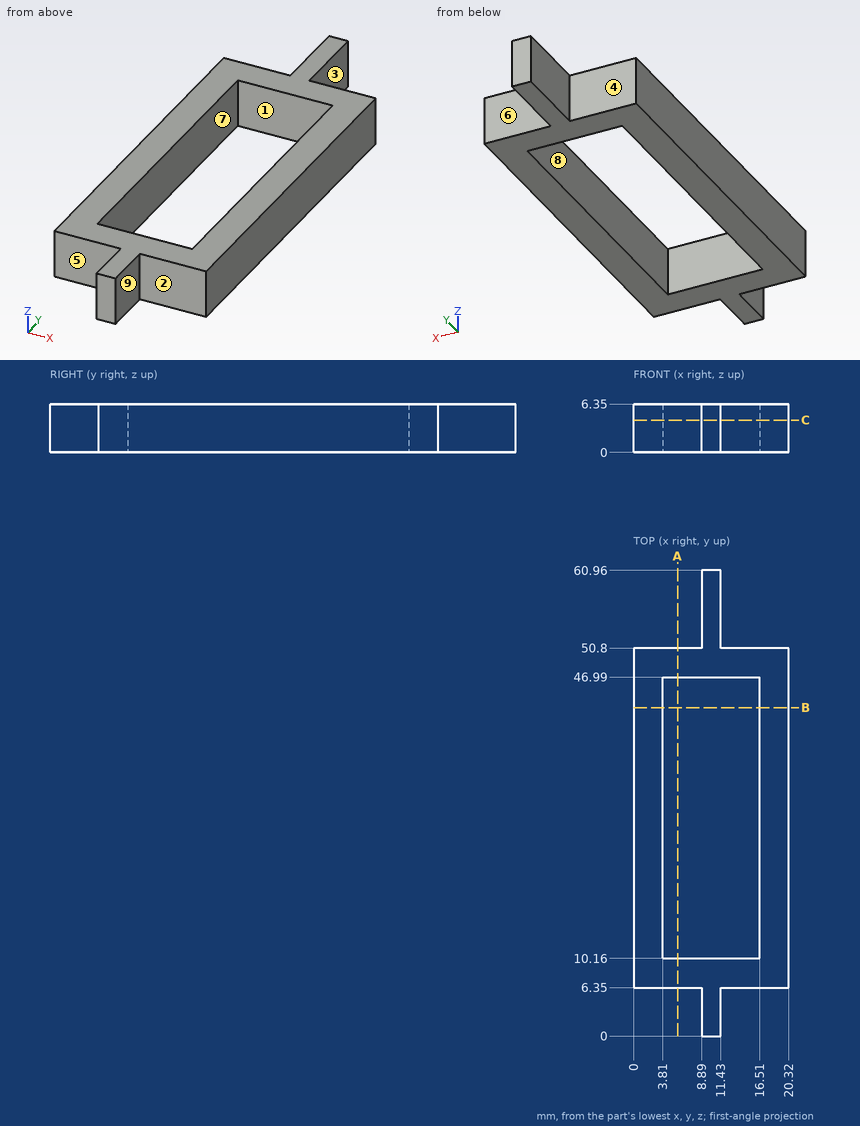
Drawing for the job (mm, zero at the part's lowest x, y, z). A direction names the side the tool comes from. Round coordinates to 2 decimals unless told otherwise and drop trailing zeros. Loops run counter-clockwise (first coordinate to the right, second up) from the corner with the lowest first, then second, coordinate; pieces in that order, holes last. Notation, with made-up numbers: (40, -33.75) -> (44, -33.75) arc R15 cw to (44, -7.75) -> close; hole circle Ø1 at (26.25, 36.5). An arc over 180 degrees is marked (long way). Answer in a Markdown table with one row per item.
Item 1: Saw through at A-A (x = 5.75). Write the cut outline in (y, z), and give its area (3 significant figures).
Answers below:
| item | result |
|---|---|
| outline | (6.35, 0) -> (10.16, 0) -> (10.16, 6.35) -> (6.35, 6.35) -> close; (46.99, 0) -> (50.8, 0) -> (50.8, 6.35) -> (46.99, 6.35) -> close |
| area | 48.4 mm² |
Item 2: Which spindle directions (+Z, -Z, +X, -X, +Y, -Y) get a long thin tool onto all of the face, cutting with end or side? Do the marked faces 1, 2, 3, 4 and 5. Say none if no direction does.
Answers below:
| item | result |
|---|---|
| face 1 | +Z, -Z |
| face 2 | +Z, -Z, +X, -Y |
| face 3 | +Z, -Z, +X, +Y |
| face 4 | +Z, -Z, -X, +Y |
| face 5 | +Z, -Z, -X, -Y |
Item 3: Pin check, flat tips, straight feed: pin 1 (2 mm diameter, centred on x = 16, z = 1.5, fed in from +Y); pin 2 (1.9 mm diameter, centred on y = 55.5, z = 2, fed in from +X); pin 3 (12 mm diameter, centred on x = 10, y = 45, fed in from +Z); pin 4 (3 mm diameter, centred on y = 4.5, z = 3.5, fed in from -X). Stop position of each tip, or through.
Answers below:
| item | result |
|---|---|
| pin 1 | stops at y = 50.8 |
| pin 2 | stops at x = 11.43 |
| pin 3 | stops at z = 6.35 |
| pin 4 | stops at x = 8.89 |
Item 4: Saw through at B-B (y = 43). Write the cut outline in (x, z), and give its area (3 significant figures).
Answers below:
| item | result |
|---|---|
| outline | (0, 0) -> (3.81, 0) -> (3.81, 6.35) -> (0, 6.35) -> close; (16.51, 0) -> (20.32, 0) -> (20.32, 6.35) -> (16.51, 6.35) -> close |
| area | 48.4 mm² |
Item 5: Saw through at C-C (z = 4.25). Write the cut outline in (x, y).
Answers below:
| item | result |
|---|---|
| outline | (0, 6.35) -> (8.89, 6.35) -> (8.89, 0) -> (11.43, 0) -> (11.43, 6.35) -> (20.32, 6.35) -> (20.32, 50.8) -> (11.43, 50.8) -> (11.43, 60.96) -> (8.89, 60.96) -> (8.89, 50.8) -> (0, 50.8) -> close; hole (3.81, 10.16) -> (16.51, 10.16) -> (16.51, 46.99) -> (3.81, 46.99) -> close |
Item 6: Mould opens along Y. For the marked faces 6, 7, 8 and 9 say: +Y half, -Y half, draft (parallel to the pull), parting line (faces both ways), or undercut.
Answers below:
| item | result |
|---|---|
| face 6 | +Y half |
| face 7 | undercut |
| face 8 | undercut |
| face 9 | draft |
Item 7: Drill centre lines: L1, parallel to Y at x = 5.25, z = 1.75; L2, parallel to Y at x = 10.5, z = 2.5; L3, parallel to X at y = 22, z = 5.5. Where is each one in solid material? Low to high. Write a range as [from, to].
Answers below:
| item | result |
|---|---|
| L1 | y = [6.35, 10.16], [46.99, 50.8] |
| L2 | y = [0, 10.16], [46.99, 60.96] |
| L3 | x = [0, 3.81], [16.51, 20.32] |
